Source: CAD feature listing. Evaluate the final solid. Frame: model axes, mm. Face numbers are marked on the shaded views. A direction names the side the tool comes from. Give positions to 0.01 mm unless a question says otherwise; leave off trailing zeros. Order: outer loops, then holes, each group sorted by start corner. A loop starts at its lowest first (then second) coordinate and runs counter-clockwise, first axis right, second up. Notation, with made-up numbers: M 17,-37.5 L 33,-37.5 A23 ccw 33,-3.5 Z; hole C -30.5,6.25 d1. An arc over 180 degrees is marked long. Use CSV: the item, a comma, the result in double quotes. Start each with the question number.
Item 1: Section query C-C on y = 11.5. Return loops of the section in (x, z), and give its area (3 significant figures).
Item 2: Section query A-A on z = 6. Return loops of the section in (x, y).
Item 3: Ray query, probe 1 along X at (y, z) = (-5.5, 4); probe 2 along Y at (x, z) = (0, 5); probe 3 along Z at (x, y) = (-10.5, -11.5). Return the intervals inside material, ascending. Write a range as from..to.
Item 4: Section query B-B on x = -9. Return loops of the section in (y, z).
Item 5: Access query for the marked faces 1, 2, 3 and 4. Directions: +Z, -Z, +X, -X, +Y, -Y. A direction counts if a zero-diameter tool reaches every point of the face in a straight line with its end or side. Return the directions, or none.
Item 6: First-contact query: pin 1 (4 mm diameter, centred on y = 16, z = 6.5, fed in from -X); pin 2 (4 mm diameter, centred on x = 23.5, z = 1.5, fed in from +Y); pin 3 (4 mm diameter, centred on x = -12, y = 11, fed in from +Z). Flat tips, straight axial feed; report the tip coordinate or a pass-through.
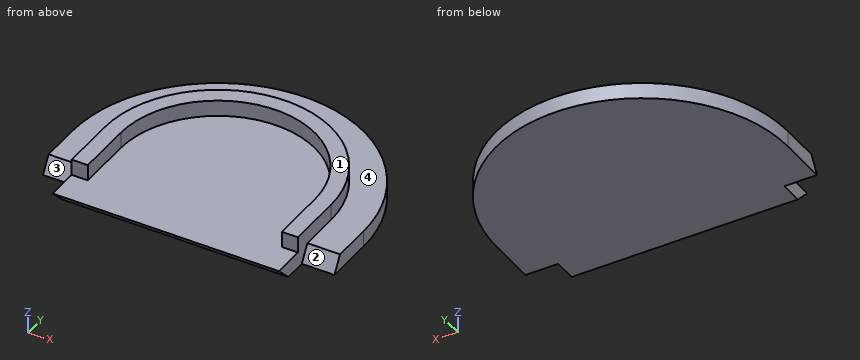
from build123d import *

# Parameters (mm, degrees)
F1_DEPTH = 3.6
F3_DEPTH = 7.3
F5_DEPTH = 7.3
F7_DEPTH = 3.6
F9_DEPTH = 57.901


with BuildPart() as f1:
    # F0 (on Top) → F1 (new body)
    with BuildSketch(Plane.XY):
        with BuildLine():
            Line((-32.6, 0), (-32.6, -11))
            Line((-32.6, -11), (-25.3, -11))
            Line((-25.3, -11), (-25.3, -21))
            Line((-25.3, -21), (25.3, -21))
            Line((25.3, -21), (25.3, -11))
            Line((25.3, -11), (32.6, -11))
            Line((32.6, -11), (32.6, 0))
            ThreePointArc((32.6, 0), (0, 32.6), (-32.6, 0))
        make_face()
    extrude(amount=F1_DEPTH)

    # F2 (on face) → F3 (cut, through all)
    with BuildSketch(Plane.YZ.offset(32.6)):
        Polygon((-8.9, 3.6), (-11, 3.6), (-11, 0), align=None)
    extrude(amount=-F3_DEPTH, mode=Mode.SUBTRACT)

    # F4 (on face) → F5 (cut, through all)
    with BuildSketch(Plane(origin=(-32.6, 0, 0), x_dir=(0, -1, 0), z_dir=(-1, 0, 0))):
        Polygon((11, 0), (11, 3.6), (8.9, 3.6), align=None)
    extrude(amount=-F5_DEPTH, mode=Mode.SUBTRACT)

    # F6 (on face) → F7 (join)
    with BuildSketch(Plane.XY.offset(3.6)):
        with BuildLine():
            Line((-25.3, 0), (-25.3, -12.5))
            Line((-25.3, -12.5), (-21.7, -12.5))
            Line((-21.7, -12.5), (-21.7, 0))
            ThreePointArc((-21.7, 0), (0, 21.7), (21.7, 0))
            Line((21.7, 0), (21.7, -12.5))
            Line((21.7, -12.5), (25.3, -12.5))
            Line((25.3, -12.5), (25.3, 0))
            ThreePointArc((25.3, 0), (0, 25.3), (-25.3, 0))
        make_face()
    extrude(amount=F7_DEPTH)

    # F8 (on face) → F9 (cut, through all)
    with BuildSketch(Plane.YZ.offset(25.3)):
        Polygon((-19.691169, 3.6), (-21, 3.6), (-21, 0), (-16.091169, 0), align=None)
    extrude(amount=-F9_DEPTH, mode=Mode.SUBTRACT)


solid = f1.part
Verdict:
1,outline,"M -30.5,0 L 30.5,0 L 30.5,3.6 L 22.54,3.6 L 22.54,7.2 L 18.4,7.2 L 18.4,3.6 L -18.4,3.6 L -18.4,7.2 L -22.54,7.2 L -22.54,3.6 L -30.5,3.6 Z"
1,area,"249 mm2"
2,outline,"M -25.3,-12.5 L -21.7,-12.5 L -21.7,0 A21.7 cw 21.7,0 L 21.7,-12.5 L 25.3,-12.5 L 25.3,0 A25.3 ccw -25.3,0 Z"
3,probe 1,"-25.3..-21.7, 21.7..25.3"
3,probe 2,"21.7..25.3"
3,probe 3,"0..3.6"
4,outline,"M -19.69,3.6 L -16.09,0 L 31.33,0 L 31.33,3.6 L 23.65,3.6 L 23.65,7.2 L 19.75,7.2 L 19.75,3.6 Z"
5,face 1,"+Z, +X, -X, +Y, -Y"
5,face 2,"+Z, +X, -Y"
5,face 3,"+Z, -X, -Y"
5,face 4,"+Z, +Y"
6,pin 1,"x = -21.07"
6,pin 2,"y = 24.51"
6,pin 3,"z = 3.6"
